The listing builds one solid part. Answer for the finished solid, in the listing's coordinates (mm). Give positions to 0.01 mm unless a question says otherwise; leave off trailing zeros. Write each loop counter-clockwise with the first axis right and the second up, starting at its lowest first coordinate (ties: lowest second). Pieces come first, ordered by that corner, then holes. Notation, with made-up numbers: (29, 3) -> (65, 3) arc R30 ccw to (65, 30) -> close; hole circle Ø1 at (-33.5, 63.25). An arc over 180 degrees is marked (long way). Put each result on its own line as item: value. Start each with the question number.
1) A cutting plane is placed at C-C (y = -24). Write down the section's boundary in (x, z) (3 decimals).
2) Flat-ended cylindrical pins translate along their axes: pin 1 Ø1 at (x, y) = (3, -13.5) entering from -Z; pin 2 Ø10 at (y, z) = (0, 0) entering from +X; pin 3 Ø8 at (y, z) = (-3.5, -8.5) entering from -X. Find the tip coordinate at first contact, or state that the pin passes through.
3) A cutting plane is placed at D-D (z = 187). Write down the section's boundary in (x, y) (3 decimals).
4) For a pull along Y with two mould halves and no side action, classify faces 1 (the cylindrical face through (2, 0, -127)), 2 (the cylindrical face through (1.57, 0.95, -117.33)), 3 (the flat face through (0, -1, 53)) as released by +Y, released by -Y, zero draft, split by the parting line, or undercut.
5) A cutting plane is placed at A-A (x = 2.35). Write down the section's boundary in (y, z) (3 decimals).
6) Find the intervals of material crossed by line 1 along Y through (x, z) = (2.55, 0); line 2 along Y through (x, z) = (0.75, -114.3) (3 decimals); line 3 along Y through (x, z) = (0.9, 187), in increasing order. Write a range as from..to.
7) A cutting plane is placed at B-B (z = 0). Write down the section's boundary in (x, y) (3 decimals).
from build123d import *

# Parameters (mm, degrees)
SKETCH1_R           = 6.35
SKETCH1_R_2         = 3.175
BOSS_EXTRUDE1_DEPTH = 3.175


with BuildPart() as part:
    # Sketch1 → Boss-Extrude1 (new body)
    # profile 1 of 2: a face of its own
    with BuildSketch(Plane.YZ):
        Polygon((0, 228.6), (-38.1, 127), (-38.1, -76.2), (-16.334358657, -111.904101294), (-12.7, -97.366666667), (12.7, -97.366666667), (16.334358657, -111.904101294), (38.1, -76.2), (38.1, 127), align=None)
        with Locations(Location((0, 0, 0), (0, 0, 270))):
            Circle(SKETCH1_R, mode=Mode.SUBTRACT)
    # profile 2 of 2: a face of its own
    with BuildSketch(Plane.YZ):
        with BuildLine():
            Line((-12.7, -97.366666667), (-16.334358657, -111.904101294))
            Line((-16.334358657, -111.904101294), (-10.843906908, -120.910573574))
            ThreePointArc((-10.843906908, -120.910573574), (0, -127), (10.843906908, -120.910573574))
            Line((10.843906908, -120.910573574), (16.334358657, -111.904101294))
            Line((16.334358657, -111.904101294), (12.7, -97.366666667))
            Line((12.7, -97.366666667), (-12.7, -97.366666667))
        make_face()
        with Locations(Location((0, -114.3, 0), (0, 0, 270))):
            Circle(SKETCH1_R_2, mode=Mode.SUBTRACT)
    extrude(amount=BOSS_EXTRUDE1_DEPTH)


solid = part.part
Reply:
1. outline: (0, -99.329) -> (3.175, -99.329) -> (3.175, 164.6) -> (0, 164.6) -> close
2. pin 1: stops at z = -117.37
2. pin 2: passes through
2. pin 3: stops at x = 0
3. outline: (0, -15.6) -> (3.175, -15.6) -> (3.175, 15.6) -> (0, 15.6) -> close
4. face 1: split by the parting line
4. face 2: undercut
4. face 3: zero draft
5. outline: (-38.1, -76.2) -> (-10.844, -120.911) arc R12.7 ccw to (10.844, -120.911) -> (38.1, -76.2) -> (38.1, 127) -> (0, 228.6) -> (-38.1, 127) -> close; hole circle Ø12.7 at (0, 0); hole circle Ø6.35 at (0, -114.3)
6. line 1: y = -38.1..-6.35, 6.35..38.1
6. line 2: y = -14.874..-3.175, 3.175..14.874
6. line 3: y = -15.6..15.6
7. outline: (0, -38.1) -> (3.175, -38.1) -> (3.175, -6.35) -> (0, -6.35) -> close; (0, 6.35) -> (3.175, 6.35) -> (3.175, 38.1) -> (0, 38.1) -> close
